Verification items for the finished model (mm, model axes). Give positions to 0.01 mm unless a question says otherwise; leave off trailing zeros. Loops run counter-clockwise (first coordinate to the right, second up) from the corner with the lowest first, then second, coordinate; pieces in that order, holes last. Notation, with made-up numbers: (3, 15.25) - (62, 15.25) arc R21 ccw to (62, 36.25) - close; hole circle Ø11 at (-31.75, 61.5). An arc over 180 degrees is marked (long way). One line per question, with ' | ' between items. Start each with the question number.
1. Section check C-C, the plane y = 12.7. Enter the section's corners in (x, z) (3 decimals), then the cut area to 3 significant figures.
2. Section check D-D, the plane x = 12.7. Enter the section's corners in (y, z) (3 decimals), then the cut area to 3 significant figures.
3. Section check A-A, the plane x = 241.3. Enter the section's corners in (y, z) (3 decimals), then the cut area to 3 significant figures.
4. Section check B-B, the plane z = 2.75. Enter the section's corners in (x, y) (3 decimals), then the cut area to 3 significant figures.
5. Thickness scan on line 1 along Y through (x, z) = (241.3, 5.25) (3 decimals); line 2 along Y through (x, z) = (12.7, 2) (3 decimals); line 3 along X through (y, z) = (10.75, 2). Record the ranges inside material, lowest first. Write a range as from..to.
from build123d import *

# Parameters (mm, degrees)
F0_W     = 254
F0_H     = 6.35
F1_DEPTH = 25.4
F2_R     = 6.985
F2_R_2   = 3.175
F3_DEPTH = 25.4
F4_R     = 5.08


with BuildPart() as f1:
    # F0 (on Front) → F1 (new body)
    with BuildSketch(Plane.XZ):
        with Locations((127, 3.175)):
            Rectangle(F0_W, F0_H)
    extrude(amount=-F1_DEPTH)

    # F2 (on face) → F3 (cut)
    with BuildSketch(Plane.XY.offset(6.35)):
        with Locations((12.7, 12.7)):
            Circle(F2_R)
        with Locations((241.3, 12.7)):
            Circle(F2_R_2)
    extrude(amount=-F3_DEPTH, mode=Mode.SUBTRACT)

    # F4
    f4_edges = [f1.edges().sort_by_distance(p)[0] for p in [
        (254, 0, 3.175),
        (254, 25.4, 3.175),
        (0, 0, 3.175),
        (0, 25.4, 3.175),
    ]]
    fillet(f4_edges, radius=F4_R)


solid = f1.part
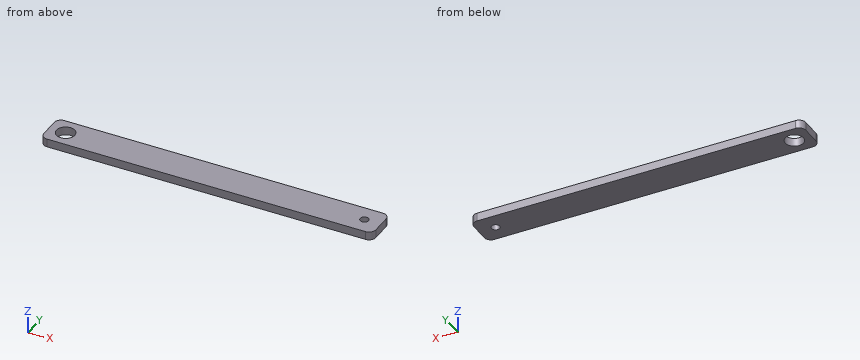
Results list:
1) outline: (0, 0) - (5.715, 0) - (5.715, 6.35) - (0, 6.35) - close; (19.685, 0) - (238.125, 0) - (238.125, 6.35) - (19.685, 6.35) - close; (244.475, 0) - (254, 0) - (254, 6.35) - (244.475, 6.35) - close | area: 1,480 mm²
2) outline: (0, 0) - (5.715, 0) - (5.715, 6.35) - (0, 6.35) - close; (19.685, 0) - (25.4, 0) - (25.4, 6.35) - (19.685, 6.35) - close | area: 72.6 mm²
3) outline: (0, 0) - (9.525, 0) - (9.525, 6.35) - (0, 6.35) - close; (15.875, 0) - (25.4, 0) - (25.4, 6.35) - (15.875, 6.35) - close | area: 121 mm²
4) outline: (0, 5.08) arc R5.08 ccw to (5.08, 0) - (248.92, 0) arc R5.08 ccw to (254, 5.08) - (254, 20.32) arc R5.08 ccw to (248.92, 25.4) - (5.08, 25.4) arc R5.08 ccw to (0, 20.32) - close; hole circle Ø13.97 at (12.7, 12.7); hole circle Ø6.35 at (241.3, 12.7) | area: 6,240 mm²
5) line 1: 0..9.525, 15.875..25.4 | line 2: 0..5.715, 19.685..25.4 | line 3: 0..5.99, 19.41..238.79, 243.81..254
